Check sheet for the drawn part. Datum: minimum x, y, z corner. Units: mm. Round coordinates to 2 decimals unless told otherwise and drop trailing zeros. Write each loop counter-clockwise with the first axis right and the second up, starting at its lowest first coordinate (ties: lowest second). Pieces come first, ordered by that corner, then holes.
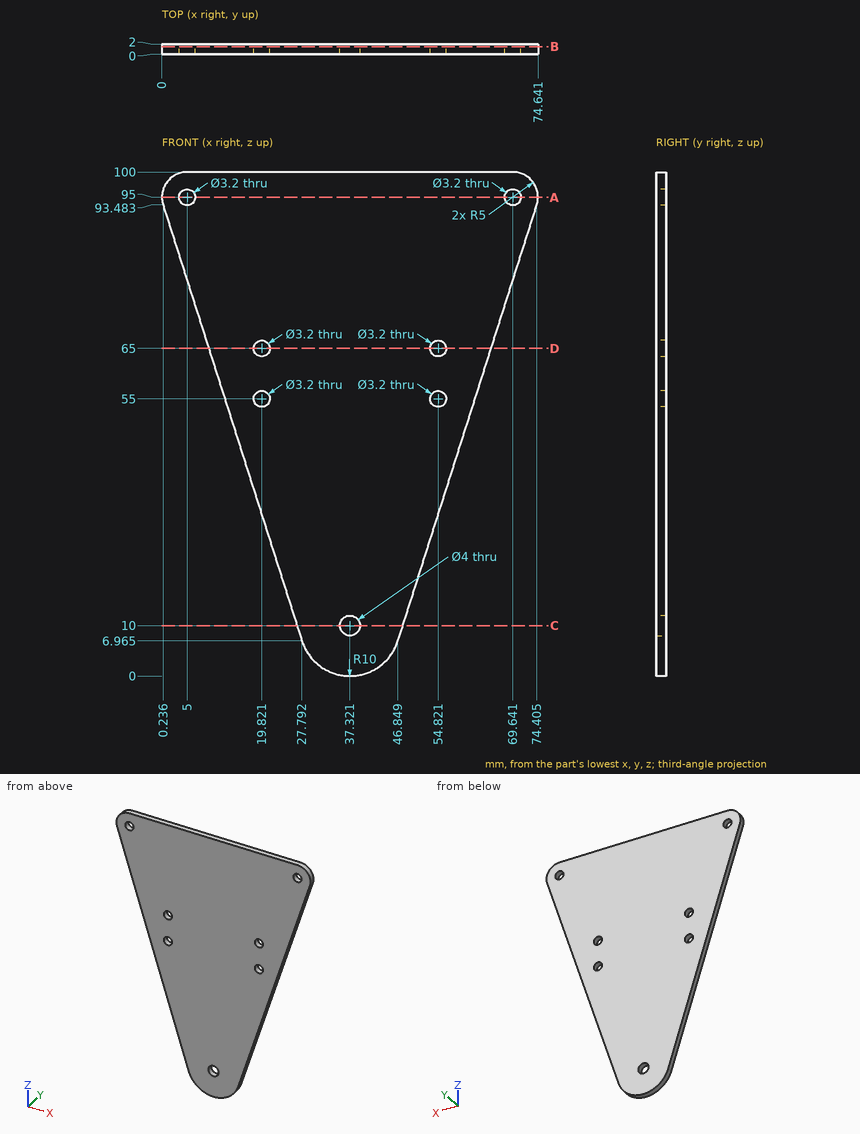
Q1. Sectioned sample at A-A (z = 95). Enter the section's corners in (x, y).
Recorded:
outline: (0, 0) - (3.4, 0) - (3.4, 2) - (0, 2) - close; (6.6, 0) - (68.04, 0) - (68.04, 2) - (6.6, 2) - close; (71.24, 0) - (74.64, 0) - (74.64, 2) - (71.24, 2) - close
Q2. Sectioned sample at B-B (y = 1.5). Enter the section's corners in (x, z) (1 decimal).
Recorded:
outline: (0.2, 93.5) - (27.8, 7) arc R10 ccw to (46.8, 7) - (74.4, 93.5) arc R5 ccw to (69.6, 100) - (5, 100) arc R5 ccw to start; hole circle Ø3.2 at (5, 95); hole circle Ø3.2 at (19.8, 55); hole circle Ø3.2 at (19.8, 65); hole circle Ø4 at (37.3, 10); hole circle Ø3.2 at (54.8, 55); hole circle Ø3.2 at (54.8, 65); hole circle Ø3.2 at (69.6, 95)
Q3. Sectioned sample at D-D (z = 65). Enter the section's corners in (x, y).
Recorded:
outline: (9.31, 0) - (18.22, 0) - (18.22, 2) - (9.31, 2) - close; (21.42, 0) - (53.22, 0) - (53.22, 2) - (21.42, 2) - close; (56.42, 0) - (65.33, 0) - (65.33, 2) - (56.42, 2) - close
Q4. Sectioned sample at C-C (z = 10). Enter the section's corners in (x, y) (1 decimal).
Recorded:
outline: (26.8, 0) - (35.3, 0) - (35.3, 2) - (26.8, 2) - close; (39.3, 0) - (47.8, 0) - (47.8, 2) - (39.3, 2) - close
Q5. Depth check by flat-ended pin: P1, Ø5, axis at x = 15, z = 35.5, coming from the -Y side; P2, Ø1, axis at x = 45, y = 1, coming from the -Z side. Enter the tip coordinate at first touch or a pass-through.
Recorded:
P1: passes through
P2: stops at z = 3.04
Q6. Material ranges on line 1 along X through (y, z) = (1.1, 95); line 2 along X through (y, z) = (1, 65); line 3 along X through (y, z) = (1.65, 10) (1 decimal), recorded low to high.
Recorded:
line 1: x = 0 to 3.4, 6.6 to 68.04, 71.24 to 74.64
line 2: x = 9.31 to 18.22, 21.42 to 53.22, 56.42 to 65.33
line 3: x = 26.8 to 35.3, 39.3 to 47.8
